For this review, use the dimensioned drawing (mm, ordinates from the lowest corner) and the shaded views. A direction names the side the tool comes from. Give positions to 0.01 mm unless a question says otherwise; leave off trailing zeros. Write each loop counter-clockwise with the first axis right and the second up, starting at its lowest first coordinate (ties: lowest second). Pieces come first, ordered by that corner, then holes. Notation, with made-up numbers: (22, 17) -> (72, 17) arc R9 cw to (72, 33) -> close; hole circle Ø4 at (16.25, -23). An arc over 180 degrees is marked (long way). Write each question's results on one line, items separated by ' | '. Start each with the question number.
(1) Take a section at C-C (y = 11.5). Count the separate pieces of the cut face and the enclosed holes in it, plus the area to 4 significant figures.
(2) Take a section at B-B (z = 10). State the section outline as (x, y) points, plus the area to 3 significant figures.
(3) To check wall thickness, follow probe 1 along Z at (x, y) = (6.75, 7); probe 2 along Y at (x, z) = (2.5, 2.5). State the ranges of each line that lie inside material, in increasing order.
(4) Clearance check with flat-ended pins moving along their axes: pin 1 (0.8 mm diameter, centred on x = 4, y = 6.5, fed in from +Z); pin 2 (1.6 mm diameter, centred on y = 7.5, z = 6.5, fed in from +X). State where each tip first meets the part, or that it passes through.
(5) Take a section at D-D (z = 7.75). State the section outline as (x, y) points, plus the area to 3 significant figures.
(6) For the marked faces 1 and 2, list the 3-axis set-ups (+Z, -Z, +X, -X, +Y, -Y) from which the entire face can be reached by the end or side of a thin tool; tool diameter is ignored.
(7) Take a section at A-A (x = 9.5). State the section outline as (y, z) points, plus the area to 3 significant figures.
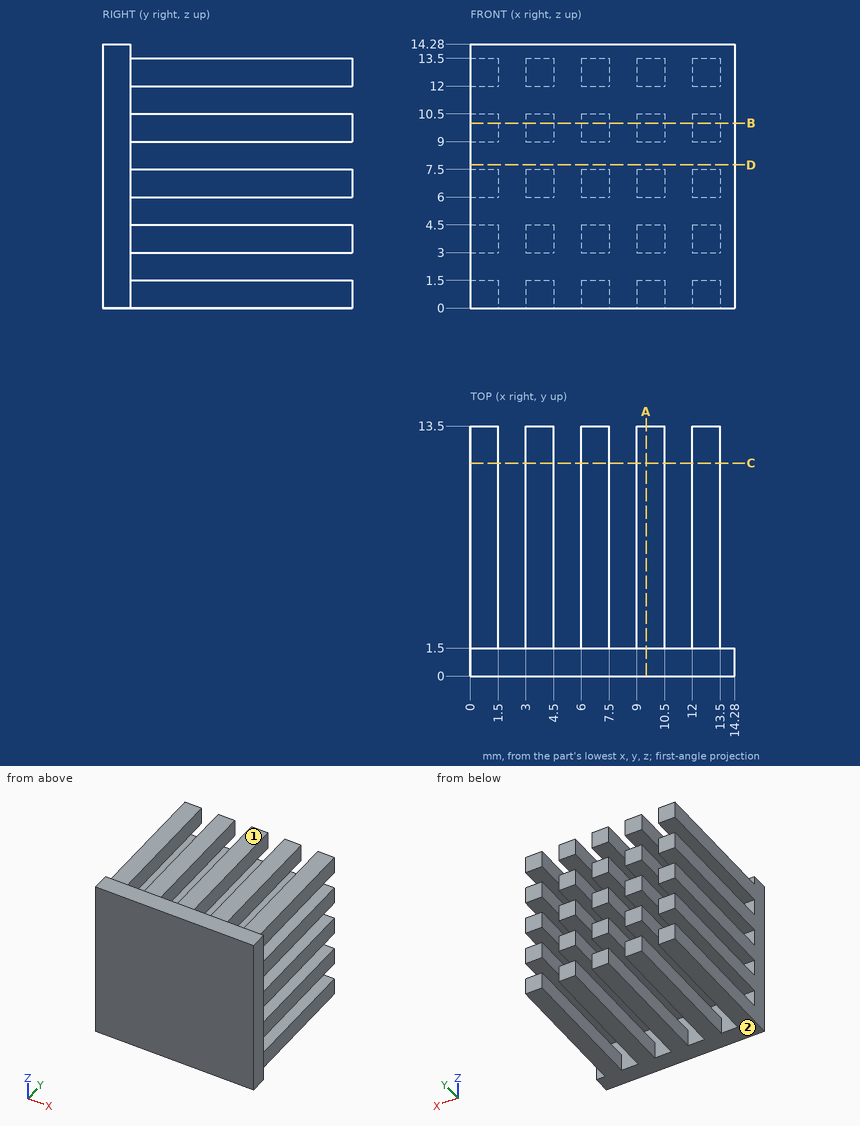
Report:
1) separate pieces: 25 | enclosed holes: 0 | area: 56.25 mm2
2) outline: (0, 0) -> (14.28, 0) -> (14.28, 1.5) -> (13.5, 1.5) -> (13.5, 13.5) -> (12, 13.5) -> (12, 1.5) -> (10.5, 1.5) -> (10.5, 13.5) -> (9, 13.5) -> (9, 1.5) -> (7.5, 1.5) -> (7.5, 13.5) -> (6, 13.5) -> (6, 1.5) -> (4.5, 1.5) -> (4.5, 13.5) -> (3, 13.5) -> (3, 1.5) -> (1.5, 1.5) -> (1.5, 13.5) -> (0, 13.5) -> close | area: 111 mm2
3) probe 1: 0 to 1.5, 3 to 4.5, 6 to 7.5, 9 to 10.5, 12 to 13.5 | probe 2: 0 to 1.5
4) pin 1: z = 13.5 | pin 2: x = 13.5
5) outline: (0, 0) -> (14.28, 0) -> (14.28, 1.5) -> (0, 1.5) -> close | area: 21.4 mm2
6) face 1: +Z, +X, -X, +Y | face 2: -Z, +X, -X, +Y, -Y
7) outline: (0, 0) -> (13.5, 0) -> (13.5, 1.5) -> (1.5, 1.5) -> (1.5, 3) -> (13.5, 3) -> (13.5, 4.5) -> (1.5, 4.5) -> (1.5, 6) -> (13.5, 6) -> (13.5, 7.5) -> (1.5, 7.5) -> (1.5, 9) -> (13.5, 9) -> (13.5, 10.5) -> (1.5, 10.5) -> (1.5, 12) -> (13.5, 12) -> (13.5, 13.5) -> (1.5, 13.5) -> (1.5, 14.28) -> (0, 14.28) -> close | area: 111 mm2
